Can you work these out from the drawing? Everything is in mm from the part's minimum corner. Coordinates: 2 decimals unless noted, no trailing zeros. Order: outer loops, then holes, each group sorted by start corner. A loop starts at its lowest first (then second) coordinate and runs counter-clockwise, first axis right, second up. Notation, with made-up numbers: (61, 54) - (117, 54) arc R19 cw to (117, 76) - close; hole circle Ø11 at (74.25, 71). An arc over 180 degrees is marked (long way). Answer as CSV lines item,"result". Start each with the question number.
Q1. Suppose I cut it at C-C (x = 0.4). Please give me the cut outline in (y, z).
Q2. Suppose I cut it at D-D (x = 4.25). Please give me the cut outline in (y, z) (1 decimal).
Q3. I need wall thicknesses on line 1 (Y direction, x = 3.9, z = 3.6); line 2 (Z direction, x = 3, y = 1.5) (1 decimal); line 3 (Y direction, x = 1.75, z = 2.6). Which ranges of each line are inside material? Lowest first, please.
Q4. Suppose I cut it at A-A (y = 0.75). Please give me the cut outline in (x, z) (1 decimal), then the cut area to 3 significant figures.
Q5. Thinking about a two-plate mould opening in Z: for the marked faces 1, 2, 3 and 4, which applies, released by +Z, released by -Z, zero draft, split by the parting line, or undercut?
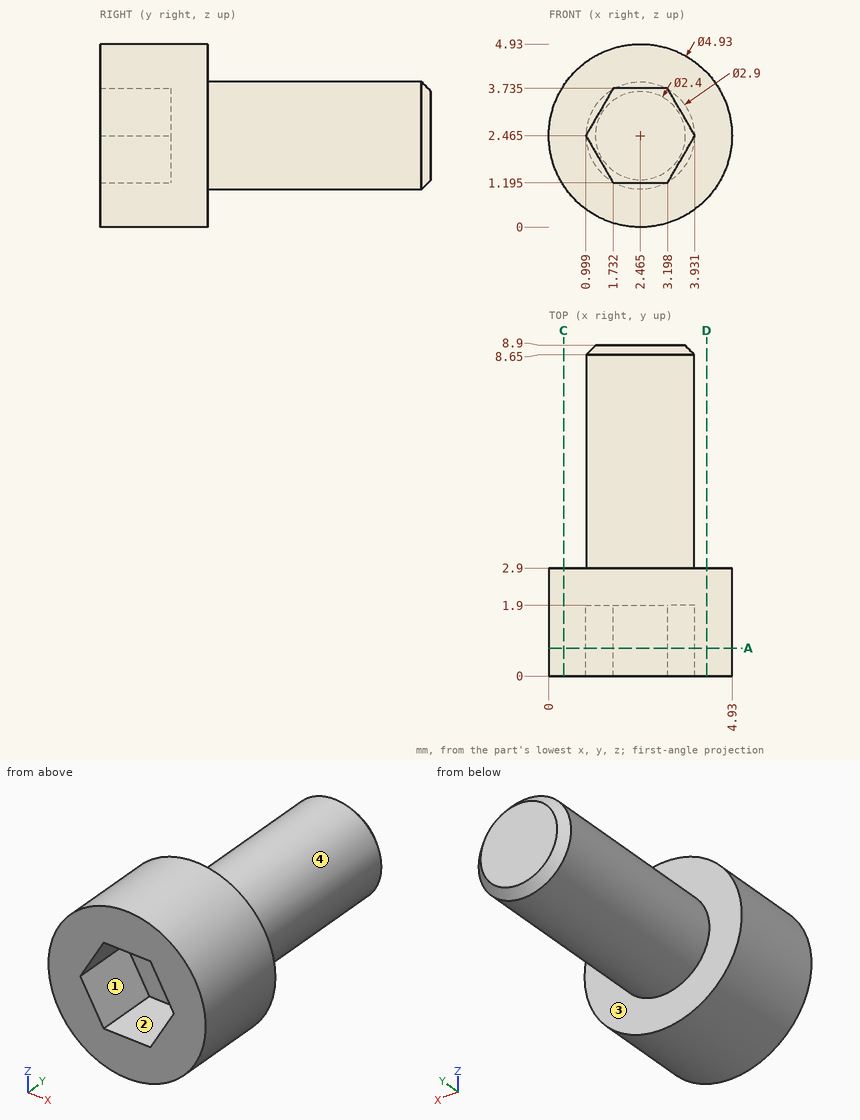
Here are the results:
1,outline,"(0, 1.12) - (2.9, 1.12) - (2.9, 3.81) - (0, 3.81) - close"
2,outline,"(0, 0.8) - (2.9, 0.8) - (2.9, 4.2) - (0, 4.2) - close"
3,line 1,"y = 0 to 2.9"
3,line 2,"z = 0.1 to 1.2, 3.7 to 4.9"
3,line 3,"y = 1.9 to 8.9"
4,outline,"circle Ø4.9 at (2.5, 2.5); hole (1, 2.5) - (1.7, 1.2) - (3.2, 1.2) - (3.9, 2.5) - (3.2, 3.7) - (1.7, 3.7) - close"
4,area,"13.5 mm²"
5,face 1,"undercut"
5,face 2,"undercut"
5,face 3,"zero draft"
5,face 4,"split by the parting line"
